```python
from build123d import *

# Parameters (mm, degrees)
EXTRUDE_1_DEPTH     = 49
SKETCH_2_W          = 8
SKETCH_2_H          = 17
CUT_EXTRUDE_1_DEPTH = 10
SKETCH_3_R          = 9
CUT_EXTRUDE_2_DEPTH = 2
FILLET_1_R          = 1
SKETCH_4_R          = 4.75
CUT_EXTRUDE_4_DEPTH = 40
SKETCH_5_W          = 4
SKETCH_5_H          = 10
CUT_EXTRUDE_5_DEPTH = 38
SKETCH_6_W          = 4
SKETCH_6_H          = 1
EXTRUDE_2_DEPTH     = 27.498032825


with BuildPart() as part:
    # 草图1 → 凸台-拉伸1 (new body)
    with BuildSketch(Plane.XZ.offset(-30.01474584)):
        with BuildLine():
            Line((43.696678655, -16.841019134), (-0.803321345, -16.841019134))
            ThreePointArc((-0.803321345, -16.841019134), (-2.217534907, -17.426805571), (-2.803321345, -18.841019134))
            Line((-2.803321345, -18.841019134), (-2.803321345, -28.341019134))
            ThreePointArc((-2.803321345, -28.341019134), (-2.217534907, -29.755232696), (-0.803321345, -30.341019134))
            Line((-0.803321345, -30.341019134), (43.696678655, -30.341019134))
            ThreePointArc((43.696678655, -30.341019134), (45.110892218, -29.755232696), (45.696678655, -28.341019134))
            Line((45.696678655, -28.341019134), (45.696678655, -18.841019134))
            ThreePointArc((45.696678655, -18.841019134), (45.110892218, -17.426805571), (43.696678655, -16.841019134))
        make_face()
    extrude(amount=EXTRUDE_1_DEPTH)

    # 草图2 → 切除-拉伸1 (cut)
    with BuildSketch(Plane.XY.offset(-16.841019134)):
        with Locations((36.643304361, -5.983286986)):
            Rectangle(SKETCH_2_W, SKETCH_2_H)
    extrude(amount=-CUT_EXTRUDE_1_DEPTH, mode=Mode.SUBTRACT)

    # 草图3 → 切除-拉伸2 (cut)
    with BuildSketch(Plane.XY.offset(-16.841019134)):
        with Locations((21.643304361, -5.983286986)):
            Circle(SKETCH_3_R)
    extrude(amount=-CUT_EXTRUDE_2_DEPTH, mode=Mode.SUBTRACT)

    # 圆角1
    fillet_1_edges = [part.edges().sort_by_distance(p)[0] for p in [
        (12.643304361, -5.983286986, -18.841019134),
        (12.643304361, -5.983286986, -16.841019134),
    ]]
    fillet(fillet_1_edges, radius=FILLET_1_R - 0.0001)  # a hair under: the kernel refuses the full size

    # 草图4 → 切除-拉伸4 (cut)
    with BuildSketch(Plane(origin=(0, 30.01474584, 0), x_dir=(1, 0, 0), z_dir=(0, 1, 0))):
        with Locations(Location((21.696678655, 24.341019134, 0), (0, 0, 270))):
            Circle(SKETCH_4_R)
    extrude(amount=-CUT_EXTRUDE_4_DEPTH, mode=Mode.SUBTRACT)

    # 草图5 → 切除-拉伸5 (cut)
    with BuildSketch(Plane(origin=(0, 30.01474584, 0), x_dir=(1, 0, 0), z_dir=(0, 1, 0))):
        with Locations((36.643304361, 21.841019134)):
            Rectangle(SKETCH_5_W, SKETCH_5_H)
    extrude(amount=-CUT_EXTRUDE_5_DEPTH, mode=Mode.SUBTRACT)

    # 草图6 → 凸台-拉伸2 (add)
    with BuildSketch(Plane(origin=(0, 30.01474584, 0), x_dir=(1, 0, 0), z_dir=(0, 1, 0))):
        with Locations((36.643304361, 26.341019134)):
            Rectangle(SKETCH_6_W, SKETCH_6_H)
    extrude(amount=-EXTRUDE_2_DEPTH)


solid = part.part
```
Can you work these out from the model? Positions are in its coordinate system, mm. A direction names the side the tool comes from. Round coordinates to 2 decimals unless told otherwise and drop trailing zeros. Loops run counter-clockwise (first coordinate to the right, second up) from the corner with the lowest first, then second, coordinate; pieces in that order, holes last.
Item 1: Suppose I cut it at C-C, the plane z = -27.75. Write out the boundary of the cut face in (x, y), then the cut area to 3 significant figures.
Item 2: If we mould it in two halves opening along X, with no side actions, what happens to faces 1 (the flat face through (16, 30.015, -24)), 2 (the flat face through (32.643, -6, -22)), 3 (the flat face through (45.697, 6, -24)), 4 (the cylindrical face through (-2.2, 5.86, -17.41))? For each: +X half, -X half, draft (parallel to the pull), parting line (faces both ways), or undercut.
Item 3: Will these pins go through, and if not, where does the flat tip stop? pin 1 Ø8 at (x, y) = (20, -3) entering from +Z; pin 2 Ø6.5 at (x, y) = (36, -2.5) entering from +Z.
Item 4: Please list where these lines run through material, in increasing order: L1, parallel to X at y = -5, z = -19.5; L2, parallel to X at y = 17.5, z = -22; L3, parallel to X at y = 18.5, z = -25.25.
Item 5: Suppose I cut it at A-A, the plane z = -23. Write out the boundary of the cut face in (x, y).
Item 6: Suppose I cut it at B-B, the plane y = 8.5. Write out the boundary of the cut face in (x, z), then the cut area to 3 significant figures.
Item 7: Which directions (+Z, -Z, +X, -X, +Y, -Y) give clear straight access to the entire face, cutting with the end or side of a thin tool? Please do faces 5 (the cylindrical face through (-2.23, 5.86, -29.74)), 6 (the flat face through (22, -9.985, -24)), 7 (the flat face through (22, -6, -18.841)), 8 (the flat face through (37, 16, -25.841)).
Reported:
1. outline: (-2.8, -18.99) - (45.7, -18.99) - (45.7, 30.01) - (25, 30.01) - (25, -9.99) - (18.39, -9.99) - (18.39, 30.01) - (-2.8, 30.01) - close
1. area: 2,110 mm2
2. face 1: draft
2. face 2: undercut
2. face 3: +X half
2. face 4: -X half
3. pin 1: stops at z = -18.84
3. pin 2: stops at z = -26.84
4. L1: x = -2.8 to 32.64, 40.64 to 45.7
4. L2: x = -2.8 to 17.56, 25.83 to 34.64, 38.64 to 45.7
4. L3: x = -2.8 to 17.03, 26.36 to 34.64, 38.64 to 45.7
5. outline: (-2.8, -18.99) - (45.7, -18.99) - (45.7, 30.01) - (38.64, 30.01) - (38.64, 2.52) - (40.64, 2.52) - (40.64, -14.48) - (32.64, -14.48) - (32.64, 2.52) - (34.64, 2.52) - (34.64, 30.01) - (26.25, 30.01) - (26.25, -9.99) - (17.14, -9.99) - (17.14, 30.01) - (-2.8, 30.01) - close
6. outline: (-2.8, -28.34) arc R2 ccw to (-0.8, -30.34) - (43.7, -30.34) arc R2 ccw to (45.7, -28.34) - (45.7, -18.84) arc R2 ccw to (43.7, -16.84) - (38.64, -16.84) - (38.64, -25.84) - (34.64, -25.84) - (34.64, -16.84) - (-0.8, -16.84) arc R2 ccw to (-2.8, -18.84) - close; hole circle Ø9.5 at (21.7, -24.34)
6. area: 544 mm2
7. face 5: -Z, -X, +Y, -Y
7. face 6: +Y
7. face 7: +Z
7. face 8: +Z, +Y
